Here's how the part is built. I have some questions about the finished solid (model axes, mm). A direction names the side the tool comes from. Round coordinates to 2 decimals unless told otherwise and drop trailing zeros. Order: outer loops, then holes, each group sorted by start corner. A loop starts at its lowest first (then second) coordinate and runs counter-clockwise, first axis right, second up.
```python
from build123d import *

# Parameters (mm, degrees)
SKETCH2_R           = 3.175
BOSS_EXTRUDE2_DEPTH = 8.89
SKETCH4_R           = 25.4
SKETCH4_R_2         = 19.05
BOSS_EXTRUDE3_DEPTH = 12.7
SKETCH4_3_R         = 41.275
SKETCH4_4_R         = 19.05
CUT_EXTRUDE1_DEPTH  = 73.955945628
CUT_EXTRUDE2_DEPTH  = 76.016052311


with BuildPart() as part:
    # Sketch2 → Boss-Extrude2 (new body)
    with BuildSketch(Plane(origin=(0, 0, 0), x_dir=(1, 0, 0), z_dir=(0, 1, 0))):
        with BuildLine():
            Line((-40.4, -50.8), (40.4, -50.8))
            ThreePointArc((40.4, -50.8), (47.753910524, -47.753910524), (50.8, -40.4))
            Line((50.8, -40.4), (50.8, 40.4))
            ThreePointArc((50.8, 40.4), (47.753910524, 47.753910524), (40.4, 50.8))
            Line((40.4, 50.8), (-40.4, 50.8))
            ThreePointArc((-40.4, 50.8), (-47.753910524, 47.753910524), (-50.8, 40.4))
            Line((-50.8, 40.4), (-50.8, -40.4))
            ThreePointArc((-50.8, -40.4), (-47.753910524, -47.753910524), (-40.4, -50.8))
        make_face()
        with Locations(Location((38.1, 38.1, 0), (0, 0, 90))):
            Circle(SKETCH2_R, mode=Mode.SUBTRACT)
        with Locations(Location((38.1, -38.1, 0), (0, 0, 90))):
            Circle(SKETCH2_R, mode=Mode.SUBTRACT)
        with Locations(Location((-38.1, -38.1, 0), (0, 0, 90))):
            Circle(SKETCH2_R, mode=Mode.SUBTRACT)
        with Locations(Location((-38.1, 38.1, 0), (0, 0, 90))):
            Circle(SKETCH2_R, mode=Mode.SUBTRACT)
    extrude(amount=BOSS_EXTRUDE2_DEPTH)

    # Sketch4 → Boss-Extrude3 (add)
    with BuildSketch(Plane(origin=(0, 8.89, 0), x_dir=(1, 0, 0), z_dir=(0, 1, 0))):
        with Locations(Location((0, 0, 0), (0, 0, 270))):
            Circle(SKETCH4_R)
        with Locations(Location((0, 0, 0), (0, 0, 270))):
            Circle(SKETCH4_R_2, mode=Mode.SUBTRACT)
    extrude(amount=BOSS_EXTRUDE3_DEPTH)

    # Sketch4_3 → section 1 of loft1
    with BuildSketch(Plane(origin=(0, 8.89, 0), x_dir=(1, 0, 0), z_dir=(0, 1, 0)), mode=Mode.PRIVATE) as loft1_s1:
        Circle(SKETCH4_3_R)
    # loft up to a face of the part (loft1)
    loft([Face(Wire([part.edges().sort_by_distance((18.515803137, 21.59, -17.387496491))[0]])), loft1_s1.sketch])

    # Sketch4_4 → Cut-Extrude1 (cut, through all)
    with BuildSketch(Plane(origin=(0, 8.89, 0), x_dir=(1, 0, 0), z_dir=(0, 1, 0))):
        with Locations(Location((0, 0, 0), (0, 0, 270))):
            Circle(SKETCH4_4_R)
    extrude(amount=CUT_EXTRUDE1_DEPTH, mode=Mode.SUBTRACT)

    # Sketch2_3 → Cut-Extrude2 (cut, through all)
    with BuildSketch(Plane(origin=(0, 0, 0), x_dir=(1, 0, 0), z_dir=(0, 1, 0))):
        with BuildLine():
            ThreePointArc((-50.8, 19.05), (-69.85, 0), (-50.8, -19.05))
            Line((-50.8, -19.05), (-50.8, 19.05))
        make_face()
        with BuildLine():
            Line((-50.8, 19.05), (-50.8, -19.05))
            ThreePointArc((-50.8, -19.05), (-37.329615818, -13.470384182), (-31.75, 0))
            ThreePointArc((-31.75, 0), (-37.329615818, 13.470384182), (-50.8, 19.05))
        make_face()
        with BuildLine():
            ThreePointArc((-19.05, 50.8), (0, 31.75), (19.05, 50.8))
            Line((19.05, 50.8), (-19.05, 50.8))
        make_face()
        with BuildLine():
            Line((-19.05, 50.8), (19.05, 50.8))
            ThreePointArc((19.05, 50.8), (0, 69.85), (-19.05, 50.8))
        make_face()
        with BuildLine():
            ThreePointArc((50.8, 19.05), (31.75, 0), (50.8, -19.05))
            Line((50.8, -19.05), (50.8, 19.05))
        make_face()
        with BuildLine():
            Line((50.8, 19.05), (50.8, -19.05))
            ThreePointArc((50.8, -19.05), (64.270384182, -13.470384182), (69.85, 0))
            ThreePointArc((69.85, 0), (64.270384182, 13.470384182), (50.8, 19.05))
        make_face()
        with BuildLine():
            ThreePointArc((-19.05, -50.8), (0, -69.85), (19.05, -50.8))
            Line((19.05, -50.8), (-19.05, -50.8))
        make_face()
        with BuildLine():
            Line((-19.05, -50.8), (19.05, -50.8))
            ThreePointArc((19.05, -50.8), (0, -31.75), (-19.05, -50.8))
        make_face()
    extrude(amount=CUT_EXTRUDE2_DEPTH, mode=Mode.SUBTRACT)


solid = part.part
```
1. If we section it at B-B, the plane x = 43.5: Write out the boundary of the cut face in (y, z), and give its area (3 significant figures).
Evaluation:
outline: (0, -50.33) - (8.89, -50.33) - (8.89, -17.6) - (0, -17.6) - close; (0, 17.6) - (8.89, 17.6) - (8.89, 50.33) - (0, 50.33) - close
area: 582 mm2
2. I'm going to push flat-ended pins straight in: P1, Ø7.5, axis at x = -38.1, z = -38.1, coming from the +Y side; P2, Ø3, axis at x = 34.5, z = -37, coming from the -Y side; P3, Ø1.5, axis at y = 12.5, z = -29, coming from the +X side; P4, Ø12, axis at x = 19.5, y = 15.5, coming from the +Z side. Where does each tip first touch, or does it pass through?
Evaluation:
P1: stops at y = 8.89
P2: stops at y = 0
P3: stops at x = 24.34
P4: stops at z = 36.06
3. If we mould it in two halves opening along Z, with no side actions, what happens to faces 4 (the cylindrical face through (-38.24, 4.38, -34.93)), 5 (the flat face through (-37, 8.89, -33)), 6 (the flat face through (-30, 4, -50.8)), 7 (the cylindrical face through (47.673, 4.383, 47.834))? For each: released by +Z, released by -Z, zero draft, split by the parting line, or undercut.
Evaluation:
face 4: undercut
face 5: zero draft
face 6: released by -Z
face 7: released by +Z
4. I need wall thicknesses on probe 1 along X at (y, z) = (4.5, -38); probe 2 along X at (y, z) = (6.75, 38.1) (3 decimals). Which ranges of each line are inside material? Lowest first, please.
Evaluation:
probe 1: x = -50.8 to -41.27, -34.93 to -14.11, 14.11 to 34.93, 41.27 to 50.8
probe 2: x = -50.8 to -41.275, -34.925 to -14.199, 14.199 to 34.925, 41.275 to 50.8
5. On a 3-axis mill with a long thin cutter (end or side, diameter ignored), from which of +Z, -Z, +X, -X, +Y, -Y can I reach the whole of each face in a straight line? I mean faces 1 (the cylindrical face through (35.954, 4.383, -35.76)), 2 (the flat face through (0, 8.89, 0)), 3 (the flat face through (-37, 8.89, 32)). Say none if no direction works.
Evaluation:
face 1: +Y, -Y
face 2: +Y
face 3: +Z, -X, +Y
